```python
from build123d import *

# Parameters (mm, degrees)
SKETCH2_W           = 38.75194
SKETCH2_H           = 24.44303
SKETCH2_R           = 1.7
BOSS_EXTRUDE1_DEPTH = 3


with BuildPart() as part:
    # Sketch2 → Boss-Extrude1 (new, symmetric)
    with BuildSketch(Plane(origin=(0, 0, 0), x_dir=(1, 0, 0), z_dir=(0, 1, 0))):
        with Locations((-1.253031638, 1.410566346)):
            Rectangle(SKETCH2_W, SKETCH2_H)
        with Locations(Location((-1.272682118, 10.954361346, 0), (0, 0, 270))):
            Circle(SKETCH2_R, mode=Mode.SUBTRACT)
        with Locations(Location((-1.277061638, -8.130948654, 0), (0, 0, 270))):
            Circle(SKETCH2_R, mode=Mode.SUBTRACT)
        Polygon((-12.629001638, 7.759051346), (11.395558827, 7.759051346), (11.395558827, 3.833946346), (13.692948362, 3.833946346), (13.692948362, -1.015843654), (11.670998362, -1.015843654), (11.670998362, -4.940948654), (-12.629001638, -4.940948654), align=None, mode=Mode.SUBTRACT)
    extrude(amount=BOSS_EXTRUDE1_DEPTH, both=True)


solid = part.part
```
Design review of the part built by this model. Coordinates are the model's own, in mm. A direction names the side the tool comes from. Coordinates: 2 decimals unless noted, no trailing zeros. Write each loop counter-clockwise with the first axis right and the second up, starting at its lowest first coordinate (ties: lowest second). Pieces come first, ordered by that corner, then holes.
1) Mouldability with a two-part tool opening along X and no side actions: class faces 3 (the flat face through (18.123, 0, -1)), 4 (the flat face through (11.396, 0, -6)), 5 (the flat face through (-6, 3, -10)) as +X half, -X half, draft (parallel to the pull), parting line (faces both ways), or undercut.
2) Add section A-A (z = 4.5). Write out the cut boundary in (x, y), plus the area to 3 significant figures.
3) Insertion check: pin 1 (2.5 mm diameter, centred on x = -1.27, z = -10.95, fed in from +Y). The pin has a flat end and moves straight along its axis. Give the tip position at first contact, or say it passes through.
4) Machinability: for faces 1 (the flat face through (13.693, 0, -1)), 2 (the flat face through (-6, -3, -10)), which of the approach directions +Z, -Z, +X, -X, +Y, -Y give a long, thin tool a straight path to every point of the face, cutting with its end or side? Answer none if there is none.
5) Add section C-C (y = -0.2). Write out the cut boundary in (x, z).
6) Add section B-B (x = 3.5). Write out the cut boundary in (y, z), plus the area to 3 significant figures.
7) To check wall thickness, follow L1, parallel to Z at x = -7.5, y = 2.15; L2, parallel to X at y = 0.95, z = 2; L3, parallel to X at y = 1.8, z = -1. State the ranges of each line that lie inside material, in increasing order.
Check result:
1. face 3: +X half
1. face 4: undercut
1. face 5: draft
2. outline: (-20.63, -3) - (-12.63, -3) - (-12.63, 3) - (-20.63, 3) - close; (11.67, -3) - (18.12, -3) - (18.12, 3) - (11.67, 3) - close
2. area: 86.7 mm2
3. pin 1: passes through
4. face 1: +Y, -Y
4. face 2: +Z, -Z, +X, -X, -Y
5. outline: (-20.63, -13.63) - (18.12, -13.63) - (18.12, 10.81) - (-20.63, 10.81) - close; hole (-12.63, -7.76) - (11.4, -7.76) - (11.4, -3.83) - (13.69, -3.83) - (13.69, 1.02) - (11.67, 1.02) - (11.67, 4.94) - (-12.63, 4.94) - close; hole circle Ø3.4 at (-1.28, 8.13); hole circle Ø3.4 at (-1.27, -10.95)
6. outline: (-3, -13.63) - (3, -13.63) - (3, -7.76) - (-3, -7.76) - close; (-3, 4.94) - (3, 4.94) - (3, 10.81) - (-3, 10.81) - close
6. area: 70.5 mm2
7. L1: z = -13.63 to -7.76, 4.94 to 10.81
7. L2: x = -20.63 to -12.63, 11.67 to 18.12
7. L3: x = -20.63 to -12.63, 13.69 to 18.12
